Input: part model. Units: mm. Frame: model coordinates. Face numbers are marked on the shaded views. A direction names the side the tool comes from. Give positions to 0.01 mm unless a question says otherwise; leave off trailing zeros. Order: outer loops, then holes, each group sorted by start corner. A loop starts at its lowest first (then second) coordinate and runs counter-clockwise, first axis right, second up. Notation, with made-up numbers: M 42,11 L 75,11 A17 cw 75,41 Z; hole C 49.25,34.5 d4. An arc over 180 degrees is marked long. Use a Markdown table: item, result.
from build123d import *

# Parameters (mm, degrees)
F1_DEPTH = 3
F3_DEPTH = 6
F5_DEPTH = 3
F7_DEPTH = 40
F9_DEPTH = 30


with BuildPart() as f1:
    # F0 (on Top) → F1 (new body)
    with BuildSketch(Plane.XY):
        with BuildLine():
            Line((-25, 0), (-5, 0))
            ThreePointArc((-5, 0), (-1.464466, 1.464466), (0, 5))
            Line((0, 5), (0, 40))
            Line((0, 40), (-30, 40))
            Line((-30, 40), (-30, 5))
            ThreePointArc((-30, 5), (-28.535534, 1.464466), (-25, 0))
        make_face()
    extrude(amount=F1_DEPTH)

    # F2 (on face) → F3 (join)
    with BuildSketch(Plane.XY.offset(3)):
        with BuildLine():
            ThreePointArc((-24, 3), (-26.12132, 3.87868), (-27, 6))
            Line((-27, 6), (-27, 40))
            Line((-27, 40), (-30, 40))
            Line((-30, 40), (-30, 5))
            ThreePointArc((-30, 5), (-28.535534, 1.464466), (-25, 0))
            Line((-25, 0), (-5, 0))
            ThreePointArc((-5, 0), (-1.464466, 1.464466), (0, 5))
            Line((0, 5), (0, 40))
            Line((0, 40), (-3, 40))
            Line((-3, 40), (-3, 6))
            ThreePointArc((-3, 6), (-3.87868, 3.87868), (-6, 3))
            Line((-6, 3), (-24, 3))
        make_face()
    extrude(amount=F3_DEPTH)

    # F4 (on face) → F5 (join)
    with BuildSketch(Plane.XY.offset(9)):
        with BuildLine():
            Line((-25, 0), (-5, 0))
            ThreePointArc((-5, 0), (-1.464466, 1.464466), (0, 5))
            Line((0, 5), (0, 40))
            Line((0, 40), (-11, 40))
            Line((-11, 40), (-11, 21))
            ThreePointArc((-11, 21), (-11.87868, 18.87868), (-14, 18))
            Line((-14, 18), (-16, 18))
            ThreePointArc((-16, 18), (-18.12132, 18.87868), (-19, 21))
            Line((-19, 21), (-19, 40))
            Line((-19, 40), (-30, 40))
            Line((-30, 40), (-30, 5))
            ThreePointArc((-30, 5), (-28.535534, 1.464466), (-25, 0))
        make_face()
    extrude(amount=F5_DEPTH)

    # F6 (on face) → F7 (join)
    with BuildSketch(Plane(origin=(0, 40, 0), x_dir=(-1, 0, 0), z_dir=(0, 1, 0))):
        Polygon((0, 0), (30, 0), (30, 3), (27, 3), (3, 3), (0, 3), align=None)
    extrude(amount=F7_DEPTH)

    # F8 (on face) → F9 (join)
    with BuildSketch(Plane(origin=(-30, 0, 0), x_dir=(0, -1, 0), z_dir=(-1, 0, 0))):
        with BuildLine():
            Line((-85, 0), (-80, 0))
            Line((-80, 0), (-80, 3))
            Line((-80, 3), (-85, 3))
            ThreePointArc((-85, 3), (-90.656854, 0.656854), (-93, -5))
            Line((-93, -5), (-93, -10))
            Line((-93, -10), (-93, -15))
            ThreePointArc((-93, -15), (-90.656854, -20.656854), (-85, -23))
            Line((-85, -23), (-80, -23))
            Line((-80, -23), (-75, -23))
            Line((-75, -23), (-75, -20))
            Line((-75, -20), (-80, -20))
            Line((-80, -20), (-85, -20))
            ThreePointArc((-85, -20), (-88.535534, -18.535534), (-90, -15))
            Line((-90, -15), (-90, -10))
            Line((-90, -10), (-90, -5))
            ThreePointArc((-90, -5), (-88.535534, -1.464466), (-85, 0))
        make_face()
    extrude(amount=-F9_DEPTH)


solid = f1.part
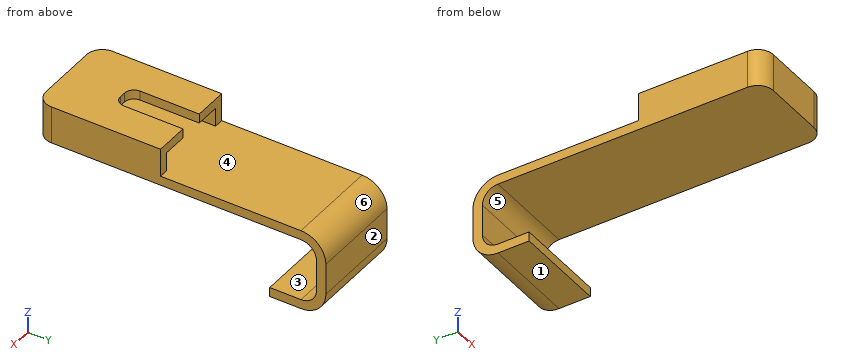
1) Cut plane C-C on x = -9. Return loops of the section in (y, z).
Response values:
| item | result |
|---|---|
| outline | M 0,0 L 85,0 A5 cw 90,-5 L 90,-15 A5 cw 85,-20 L 75,-20 L 75,-23 L 85,-23 A8 ccw 93,-15 L 93,-5 A8 ccw 85,3 L 3,3 L 3,9 L 40,9 L 40,12 L 0,12 Z |
2) Cut plane D-D on z = 4. Return loops of the section in (x, y), and give its area (3 significant figures).
Response values:
| item | result |
|---|---|
| outline | M -30,5 A5 ccw -25,0 L -5,0 A5 ccw 0,5 L 0,40 L -3,40 L -3,6 A3 cw -6,3 L -24,3 A3 cw -27,6 L -27,40 L -30,40 Z |
| area | 305 mm² |
3) First-contact query: pin 1 Ø1 at (x, z) = (-17.5, -8.5) entering from -Y; pin 2 Ø4.5 at (x, z) = (-7.5, 5.5) entering from +Y; pin 3 Ø5 at (x, z) = (-4.5, -4) entering from +Y; pin 4 Ø9 at (x, y) = (-11.5, 54) entering from -Z. Flat tips, straight axial feed; report the tip coordinate or a pass-through.
Response values:
| item | result |
|---|---|
| pin 1 | stops at y = 90 |
| pin 2 | stops at y = 3.1 |
| pin 3 | stops at y = 93 |
| pin 4 | stops at z = 0 |
4) Cut plane A-A on y = 79.5. Return loops of the section in (x, z).
Response values:
| item | result |
|---|---|
| outline | M -30,-23 L 0,-23 L 0,-20 L -30,-20 Z; M -30,0 L 0,0 L 0,3 L -30,3 Z |
5) Cut plane B-B on y = 8.5. Return loops of the section in (x, z).
Response values:
| item | result |
|---|---|
| outline | M -30,0 L 0,0 L 0,12 L -30,12 Z; hole M -27,3 L -3,3 L -3,9 L -27,9 Z |
6) Mould query, pull axis Z, two halves, no side actions, for the marked faces 1, 2 and 3. Classes: released by +Z, released by -Z, zero draft, split by the parting line, or undercut.
Response values:
| item | result |
|---|---|
| face 1 | released by -Z |
| face 2 | zero draft |
| face 3 | undercut |
7) Material intervals for line 1 (Z direction, x = -16, y = 9); line 2 (Y direction, x = -9, z = 4.5); line 3 (Z direction, x = -2, y = 14), sorted ascending. Write a range as from..to.
Response values:
| item | result |
|---|---|
| line 1 | z = 0..3, 9..12 |
| line 2 | y = 0..3 |
| line 3 | z = 0..12 |
8) Reachability of the marked faces 4, 5 and 6 from +Z, -Z, +X, -X, +Y, -Y: full face, straight path, thin tool, end or side. Return the list, or none.
Response values:
| item | result |
|---|---|
| face 4 | +Y |
| face 5 | +X, -X, -Y |
| face 6 | +Z, +X, -X, +Y |
